from build123d import *

# Parameters (mm, degrees)
BOSS_EXTRUDE1_DEPTH     = 24
SKETCH3_W               = 4
SKETCH3_H               = 35
CUT_EXTRUDE1_DEPTH      = 26.6
CUT_EXTRUDE2_DEPTH      = 31.5
CUT_EXTRUDE2_DEPTH_BACK = 31.5
SKETCH5_W               = 14
SKETCH5_H               = 61
SKETCH5_R               = 2.6
BOSS_EXTRUDE2_DEPTH     = 6
FILLET1_R               = 4
CHAMFER1_SIZE           = 1
CHAMFER2_SIZE           = 0.5


with BuildPart() as part:
    # Sketch2 → Boss-Extrude1 (new body, symmetric)
    with BuildSketch(Plane(origin=(0, 0, 0), x_dir=(0, 0, -1), z_dir=(1, 0, 0))):
        Polygon((-30.5, 35), (-22.7, 35), (-22.7, 0), (0, 0), (22.7, 0), (22.7, 35), (30.5, 35), (30.5, -6), (-30.5, -6), align=None)
    extrude(amount=BOSS_EXTRUDE1_DEPTH, both=True)

    # Sketch3 → Cut-Extrude1 (cut, symmetric)
    with BuildSketch(Plane.XY):
        with Locations((-11, 17.5)):
            Rectangle(SKETCH3_W, SKETCH3_H)
        with Locations((11, 17.5)):
            Rectangle(SKETCH3_W, SKETCH3_H)
    extrude(amount=CUT_EXTRUDE1_DEPTH, both=True, mode=Mode.SUBTRACT)

    # Sketch4 → Cut-Extrude2 (cut, two sides)
    with BuildSketch(Plane.XY) as cut_extrude2_sk:
        with BuildLine():
            Line((-16.45, 20.5), (-16.45, 6.5))
            ThreePointArc((-16.45, 6.5), (-18.5, 4.45), (-20.55, 6.5))
            Line((-20.55, 6.5), (-20.55, 20.5))
            ThreePointArc((-20.55, 20.5), (-18.5, 22.55), (-16.45, 20.5))
        make_face()
        with BuildLine():
            Line((20.55, 20.5), (20.55, 6.5))
            ThreePointArc((20.55, 6.5), (18.5, 4.45), (16.45, 6.5))
            Line((16.45, 6.5), (16.45, 20.5))
            ThreePointArc((16.45, 20.5), (18.5, 22.55), (20.55, 20.5))
        make_face()
    extrude(amount=CUT_EXTRUDE2_DEPTH, mode=Mode.SUBTRACT)
    extrude(cut_extrude2_sk.sketch, amount=-CUT_EXTRUDE2_DEPTH_BACK, mode=Mode.SUBTRACT)

    # Sketch5 → Boss-Extrude2 (add)
    with BuildSketch(Plane(origin=(0, 0, 0), x_dir=(1, 0, 0), z_dir=(0, 1, 0))):
        with Locations((-31, 0)):
            Rectangle(SKETCH5_W, SKETCH5_H)
        with Locations((-31, 23.5)):
            Circle(SKETCH5_R, mode=Mode.SUBTRACT)
        with Locations((-31, -23.5)):
            Circle(SKETCH5_R, mode=Mode.SUBTRACT)
        with Locations((31, 0)):
            Rectangle(SKETCH5_W, SKETCH5_H)
        with Locations((31, 23.5)):
            Circle(SKETCH5_R, mode=Mode.SUBTRACT)
        with Locations((31, -23.5)):
            Circle(SKETCH5_R, mode=Mode.SUBTRACT)
    extrude(amount=-BOSS_EXTRUDE2_DEPTH)

    # Fillet1
    fillet1_edges = [part.edges().sort_by_distance(p)[0] for p in [
        (-38, -3, -30.5),
        (-38, -3, 30.5),
        (38, -3, 30.5),
        (38, -3, -30.5),
    ]]
    fillet(fillet1_edges, radius=FILLET1_R)

    # Chamfer1
    chamfer1_edges = [part.edges().sort_by_distance(p)[0] for p in [
        (-24, 17.5, -22.7),
        (-24, 35, -26.6),
        (-24, 17.5, 30.5),
        (24, 35, -26.6),
        (-24, 17.5, -30.5),
        (-29, 0, -30.5),
        (0, 35, 30.5),
        (18.5, 35, 22.7),
        (24, 17.5, -30.5),
        (18.5, 35, -22.7),
        (29, 0, 30.5),
        (0, 35, -30.5),
        (24, 17.5, -22.7),
        (0, -6, -30.5),
        (29, 0, -30.5),
        (-38, 0, 0),
        (-29, 0, 30.5),
        (38, 0, 0),
        (36.828427125, 0, 29.328427125),
        (36.828427125, 0, -29.328427125),
        (-36.828427125, 0, 29.328427125),
        (-36.828427125, 0, -29.328427125),
        (-38, -6, 0),
        (0, -6, 30.5),
        (38, -6, 0),
        (36.828427125, -6, 29.328427125),
        (36.828427125, -6, -29.328427125),
        (-36.828427125, -6, 29.328427125),
        (-36.828427125, -6, -29.328427125),
        (24, 17.5, 22.7),
        (0, 35, 22.7),
        (24, 35, 26.6),
        (-18.5, 35, 22.7),
        (0, 35, -22.7),
        (-18.5, 35, -22.7),
        (24, 17.5, 30.5),
        (-11, 35, -26.6),
        (-13, 17.5, -22.7),
        (-13, 17.5, 22.7),
        (-9, 17.5, -22.7),
        (-9, 17.5, 22.7),
        (-11, 35, 26.6),
        (11, 35, -26.6),
        (9, 17.5, -22.7),
        (9, 17.5, 22.7),
        (13, 17.5, -22.7),
        (13, 17.5, 22.7),
        (11, 35, 26.6),
        (-24, 35, 26.6),
        (-24, 17.5, 22.7),
    ]]
    chamfer(chamfer1_edges, length=CHAMFER1_SIZE)

    # Chamfer2
    chamfer2_edges = [part.edges().sort_by_distance(p)[0] for p in [
        (-18.5, 22.55, 30.5),
        (-20.55, 13.5, 30.5),
        (-18.5, 4.45, 30.5),
        (-16.45, 13.5, 30.5),
        (18.5, 22.55, -22.7),
        (18.5, 22.55, -30.5),
        (20.55, 13.5, -22.7),
        (20.55, 13.5, -30.5),
        (18.5, 4.45, -22.7),
        (18.5, 4.45, -30.5),
        (16.45, 13.5, -22.7),
        (16.45, 13.5, -30.5),
        (18.5, 22.55, 30.5),
        (16.45, 13.5, 30.5),
        (18.5, 4.45, 30.5),
        (20.55, 13.5, 30.5),
        (-33.6, -6, -23.5),
        (-33.6, 0, -23.5),
        (-33.6, -6, 23.5),
        (-33.6, 0, 23.5),
        (28.4, -6, -23.5),
        (28.4, 0, -23.5),
        (28.4, -6, 23.5),
        (28.4, 0, 23.5),
        (16.45, 13.5, 22.7),
        (18.5, 4.45, 22.7),
        (20.55, 13.5, 22.7),
        (18.5, 22.55, 22.7),
        (-18.5, 22.55, -22.7),
        (-18.5, 22.55, -30.5),
        (-18.5, 22.55, 22.7),
        (-16.45, 13.5, -22.7),
        (-16.45, 13.5, -30.5),
        (-16.45, 13.5, 22.7),
        (-18.5, 4.45, -22.7),
        (-18.5, 4.45, -30.5),
        (-18.5, 4.45, 22.7),
        (-20.55, 13.5, -22.7),
        (-20.55, 13.5, -30.5),
        (-20.55, 13.5, 22.7),
    ]]
    chamfer(chamfer2_edges, length=CHAMFER2_SIZE)


solid = part.part
Read the model definition and answer for the solid it produces. Units are mm, in the model's axes. A direction names the side the tool comes from. Round coordinates to 2 decimals unless told otherwise and drop trailing zeros. Write each loop counter-clockwise with the first axis right and the second up, starting at its lowest first coordinate (ties: lowest second). Pieces come first, ordered by that corner, then holes.
1. Straight lines are drawn through the part: L1, parallel to X at y = -1.95, z = 23.5; L2, parallel to Z at x = -31, y = -3; L3, parallel to X at y = 30, z = -24. For each, find the intervals that lie inside material, in ascending order.
2. The part is cut by section C-C, the plane z = 6.5. Determine the outline of the cut face in (x, y), then the cut area to 3 significant figures.
3. Determine the mould class of faces 1 (the face through (36.348, -5.715, -28.797)), 2 (the face through (38, -3, 0)), 3 (the face through (18.55, 4.45, -26.55)), 4 (the face through (36.297, -0.285, 28.848)) for opening direction Y: pulls with the +Y half, pulls with the -Y half, needs draft (parallel to the pull), parting line crosses it, or undercut.
4. The part is cut by section D-D, the plane x = -6.5. Determine the outline of the cut face in (y, z), then the cut area to 3 significant figures.
5. Which of the six approach directions +Z, -Z, +X, -X, +Y, -Y give full straight-line access (tool end or side, diameter ignored) to faces 5 (the face through (9, 17, 25)), 6 (the face through (-18.548, 22.685, 30.135)), 7 (the face through (-18.55, 22.55, -26.55))?
6. The part is cut by section A-A, the plane x = -18.5. State how many separate pieces and enclosed holes the cut face has, then the cut area to 3 significant figures.
7. Given pin 1 Ø4.5 at (y, z) = (15.5, -26) entering from -X; pin 2 Ø4 at (x, z) = (-11.5, -5) entering from +Y; pin 3 Ø4.5 at (y, z) = (13, -26) entering from +X, each flat-ended and moving along its own axis, determine where each tip first touches the part or whether it passes through.
Values:
1. L1: x = -38 to -33.6, -28.4 to 28.4, 33.6 to 38
1. L2: z = -30.5 to -26.1, -20.9 to 20.9, 26.1 to 30.5
1. L3: x = -24 to -13, -9 to 9, 13 to 24
2. outline: (-38, -5) - (-37, -6) - (37, -6) - (38, -5) - (38, -1) - (37, 0) - (-37, 0) - (-38, -1) - close
2. area: 454 mm2
3. face 1: pulls with the -Y half
3. face 2: needs draft
3. face 3: undercut
3. face 4: pulls with the +Y half
4. outline: (-6, -29.5) - (-5, -30.5) - (34, -30.5) - (35, -29.5) - (35, -23.7) - (34, -22.7) - (0, -22.7) - (0, 22.7) - (34, 22.7) - (35, 23.7) - (35, 29.5) - (34, 30.5) - (-5, 30.5) - (-6, 29.5) - close
4. area: 909 mm2
5. face 5: +Y
5. face 6: +Z
5. face 7: +Z, -Z
6. separate pieces: 3
6. enclosed holes: 0
6. area: 626 mm2
7. pin 1: stops at x = -24
7. pin 2: stops at y = 0
7. pin 3: stops at x = 24
